Could you check a few things on this drawing? It's one solid part, dimensions in mm from its lowest x, y, z. Round coordinates to 2 decimals unless told otherwise and drop trailing zeros. Write each loop counter-clockwise with the first axis right and the second up, starting at its lowest first coordinate (ties: lowest second). Pieces come first, ordered by that corner, then holes. Notation, with made-up numbers: M 81,28 L 88,28 A11 ccw 88,35 Z; hole C 45,6 d10. An arc over 180 degrees is marked long. One line per question, with ' | ' between items. Start each with the question number.
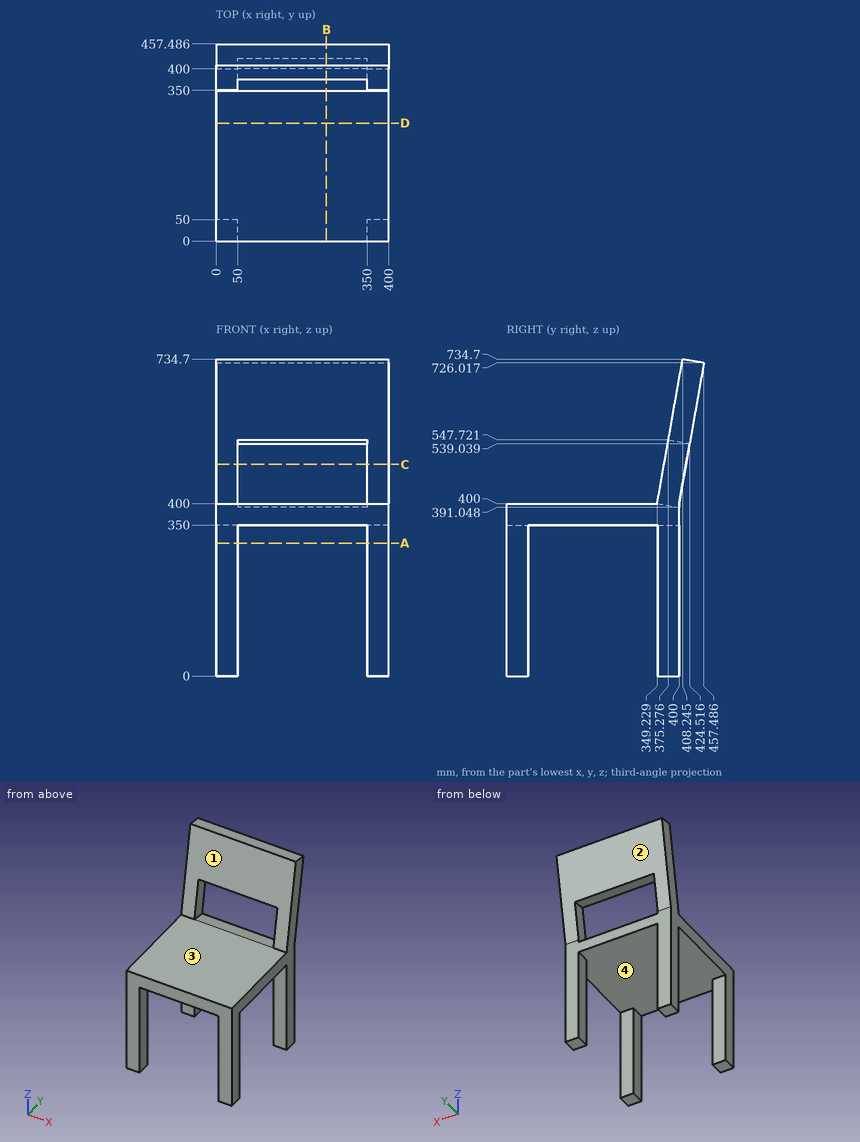
1. I need wall thicknesses on line 1 along X through (y, z) = (391.5, 93); line 2 along Z through (x, y) = (245.5, 138); line 3 along Y through (x, z) = (194, 671) (1 decimal). Which ranges of each line are inside material? Lowest first, please. Write a range as from..to.
2. I'm going to push flat-ended pins straight in: P1, Ø5, axis at x = 324, z = 647, coming from the +Y side; P2, Ø8, axis at x = 184, y = 258.5, coming from the +Z side; P3, Ø25, axis at x = 32.5, z = 96.5, coming from the +Y side. Where does each tip first touch, or does it pass through?
3. If we mould it in two halves opening along Y, with no side actions, what happens to the marked faces 1, 2, 3 and 4? For each: released by +Y, released by -Y, zero draft, split by the parting line, or undercut.
4. Suppose I cut it at C-C (z = 491). Write out the boundary of the cut face in (x, y) (1 decimal), and give its area (3 significant figures).
5. Suppose I cut it at A-A (z = 308). Write out the boundary of the cut face in (x, y), and give its area (3 significant figures).
6. Suppose I cut it at D-D (y = 274). Write out the boundary of the cut face in (x, z).
7. Suppose I cut it at B-B (x = 255.5). Write out the boundary of the cut face in (y, z) (1 decimal).
Computed:
1) line 1: x = 0..50, 350..400 | line 2: z = 350..400 | line 3: y = 397..447.8
2) P1: stops at y = 443.99 | P2: stops at z = 400 | P3: stops at y = 400
3) face 1: released by -Y | face 2: released by +Y | face 3: zero draft | face 4: undercut
4) outline: M 0,365.3 L 50,365.3 L 50,416 L 0,416 Z; M 350,365.3 L 400,365.3 L 400,416 L 350,416 Z | area: 5,080 mm²
5) outline: M 0,0 L 50,0 L 50,50 L 0,50 Z; M 0,350 L 50,350 L 50,400 L 0,400 Z; M 350,0 L 400,0 L 400,50 L 350,50 Z; M 350,350 L 400,350 L 400,400 L 350,400 Z | area: 10,000 mm²
6) outline: M 0,350 L 400,350 L 400,400 L 0,400 Z
7) outline: M 0,350 L 400,350 L 400,391 L 349.2,400 L 0,400 Z; M 375.3,547.7 L 424.5,539 L 457.5,726 L 408.2,734.7 Z
